Autodesk Inventor part; units mm, degrees
ref_plane "YZ Plane" through (0, 0, 0) normal (1, 0, 0) x (0, 1, 0)
ref_plane "XZ Plane" through (0, 0, 0) normal (0, 1, 0) x (-1, 0, 0)
ref_plane "XY Plane" through (0, 0, 0) normal (0, 0, 1) x (1, 0, 0)
sketch "スケッチ1" plane through (0, 0, 0) normal (0, 1, 0) x (-1, 0, 0)
  line L0 (41.0243, -3.6426) -> (37.5574, -0.1757)
  line L1 (41.0243, -37.5574) -> (37.5574, -41.0243)
  line L2 (3.6426, -0.1757) -> (0.1757, -3.6426)
  line L3 (0.1757, -37.5574) -> (3.6426, -41.0243)
  line L4 (0, -37.1331) -> (0, -4.0669)
  line L5 (37.1331, -41.2) -> (4.0669, -41.2)
  line L6 (41.2, -4.0669) -> (41.2, -37.1331)
  line L7 (37.1331, 0) -> (4.0669, 0)
  arc A0 (41.2, -4.0669) -> (41.0243, -3.6426) centre (40.6, -4.0669) ccw
  arc A1 (37.5574, -0.1757) -> (37.1331, 0) centre (37.1331, -0.6) ccw
  arc A2 (4.0669, 0) -> (3.6426, -0.1757) centre (4.0669, -0.6) ccw
  arc A3 (0.1757, -3.6426) -> (0, -4.0669) centre (0.6, -4.0669) ccw
  arc A4 (0, -37.1331) -> (0.1757, -37.5574) centre (0.6, -37.1331) ccw
  arc A5 (3.6426, -41.0243) -> (4.0669, -41.2) centre (4.0669, -40.6) ccw
  arc A6 (37.1331, -41.2) -> (37.5574, -41.0243) centre (37.1331, -40.6) ccw
  arc A7 (41.0243, -37.5574) -> (41.2, -37.1331) centre (40.6, -37.1331) ccw
  line L8 (25.8, 0) -> (15.4, 0)
  point P0 (0, 0)
  point P1 (41.2, -3.8184)
  point P2 (37.3816, 0)
  point P3 (39.2908, -1.9092)
  point P4 (37.3816, -41.2)
  point P5 (41.2, -37.3816)
  dimension "d2" = 5.4
  dimension "d3" = 5.4
  dimension "d4" = 0.6
extrude "押し出し1" add sketch "スケッチ1" along normal blind 9.8
sketch "スケッチ2" plane through (0, 9.8, 0) normal (0, 1, 0) x (1, 0, 0)
  line L0 (-41.2, 37.1331) -> (-41.2, 4.0669)
  line L1 (-41.0243, 3.6426) -> (-37.5574, 0.1757)
  line L2 (-4.0669, 41.2) -> (-37.1331, 41.2)
  line L3 (0, 4.0669) -> (0, 37.1331)
  line L4 (-37.1331, 0) -> (-4.0669, 0)
  line L5 (0, 34.1568) -> (0, 7.099)
  line L6 (-7.099, 0) -> (-34.1289, 0)
  line L7 (-41.2, 7.0711) -> (-41.2, 34.1568)
  line L8 (-37.5574, 41.0243) -> (-41.0243, 37.5574)
  line L9 (-3.6426, 0.1757) -> (-0.1757, 3.6426)
  arc A0 (-41.2, 7.0711) -> (-34.1289, 0) centre (-20.6, 20.6) ccw
  arc A1 (-7.071, 0) -> (0, 7.071) centre (-20.6, 20.6) ccw
  arc A2 (0, 34.1289) -> (-7.0711, 41.2) centre (-20.6, 20.6) ccw
  arc A3 (-34.1289, 41.2) -> (-41.2, 34.1289) centre (-20.6, 20.6) ccw
  line L10 (-34.1289, 0) -> (-7.071, 0)
  line L11 (-41.2, 7.0711) -> (-41.2, 34.1289)
  line L12 (-34.1289, 41.2) -> (-7.0711, 41.2)
  line L13 (0, 34.1289) -> (0, 7.071)
  point P0 (0, 0)
  point P1 (0, 40.8633)
  point P2 (-37.6645, 3.5355)
  point P3 (0, 34.1289)
  point P4 (-41.2, 41.2)
  point P5 (-7.071, 0)
  point P6 (0, 7.071)
  dimension "d8" = 10
  dimension "d9" = 10
extrude "押し出し2" add sketch "スケッチ2" along normal blind 3.8
ref_plane "作業平面1" through (0, 13.6, 0) normal (0, 1, 0) x (1, 0, 0)
sketch "スケッチ4" plane through (0, 13.6, 0) normal (0, 1, 0) x (1, 0, 0)
  line L0 (-4.0669, 0) -> (-37.1331, 0)
  line L1 (-41.2, 4.0669) -> (-41.2, 37.1331)
  line L2 (-37.1331, 41.2) -> (-4.0669, 41.2)
  line L3 (0, 37.1331) -> (0, 4.0669)
  line L4 (-41.0243, 3.6426) -> (-37.5574, 0.1757)
  line L5 (-41.0243, 3.6426) -> (-37.5574, 0.1757)
  line L6 (-0.1757, 37.5574) -> (-3.6426, 41.0243)
  line L7 (-3.6426, 41.0243) -> (-0.1757, 37.5574)
  line L8 (-3.6426, 0.1757) -> (-0.1757, 3.6426)
  line L9 (-0.1757, 3.6426) -> (-3.6426, 0.1757)
  line L10 (-37.5574, 41.0243) -> (-41.0243, 37.5574)
  line L11 (-37.5574, 41.0243) -> (-41.0243, 37.5574)
  arc A0 (-37.1331, 41.2) -> (-37.5574, 41.0243) centre (-37.1331, 40.6) ccw
  arc A1 (-41.0243, 37.5574) -> (-41.2, 37.1331) centre (-40.6, 37.1331) ccw
  line L12 (-41.0243, 3.6426) -> (-37.5574, 0.1757)
  arc A2 (-41.2, 4.0669) -> (-41.0243, 3.6426) centre (-40.6, 4.0669) ccw
  arc A3 (-37.5574, 0.1757) -> (-37.1331, 0) centre (-37.1331, 0.6) ccw
  arc A4 (-3.6426, 41.0243) -> (-4.0669, 41.2) centre (-4.0669, 40.6) ccw
  arc A5 (0, 37.1331) -> (-0.1757, 37.5574) centre (-0.6, 37.1331) ccw
  line L13 (-0.1757, 3.6426) -> (-3.6426, 0.1757)
  arc A6 (-0.1757, 3.6426) -> (0, 4.0669) centre (-0.6, 4.0669) ccw
  arc A7 (-4.0669, 0) -> (-3.6426, 0.1757) centre (-4.0669, 0.6) ccw
  point P0 (0, 0)
  point P1 (-41.2, 41.2)
  point P2 (-41.2, 0)
  point P3 (0, 41.2)
  point P4 (-41.0243, 37.5574)
  point P5 (-0.1757, 3.6426)
  dimension "d16" = 41.2
  dimension "d17" = 41.2
  dimension "d18" = 0.6
  dimension "d19" = 0.6
  dimension "d20" = 0.6
  dimension "d21" = 0.6
  dimension "d22" = 0.6
extrude "押し出し3" add sketch "スケッチ4" along normal blind 9.8
ref_plane "作業平面2" through (0, 0, 0) normal (0, -1, 0) x (1, 0, 0)
sketch "スケッチ5" plane through (0, 0, 0) normal (0, -1, 0) x (1, 0, 0)
  line L0 (-37.1331, 0) -> (-4.0669, 0)
  line L1 (-37.1331, 0) -> (-4.0669, 0)
  line L2 (-28.3, 0) -> (-12.9, 0)
  line L3 (-12.9, 0) -> (-12.9, 3.9)
  line L4 (-13, 4) -> (-28.2, 4)
  line L5 (-28.3, 3.9) -> (-28.3, 0)
  arc A0 (-28.2, 4) -> (-28.3, 3.9) centre (-28.2, 3.9) ccw
  arc A1 (-12.9, 3.9) -> (-13, 4) centre (-13, 3.9) ccw
  point P0 (0, 0)
  point P1 (-15.4, 0)
  point P2 (-12.9, 4)
  point P3 (-28.3, 4)
  point P4 (-28.3, 0)
  point P5 (-12.9, 0)
  point P6 (-20.6, 0)
  point P7 (-20.6, 0)
  dimension "d35" = 0.1
  dimension "d77" = 15.4
extrude "押し出し4" add sketch "スケッチ5" against normal blind 2
fillet "フィレット1" radius 0.1 5 edges at (-12.9, 2, 1.95) (-20.6, 2, 4) (-28.2707, 2, 3.9707) (-28.3, 2, 1.95) (-12.9293, 2, 3.9707)
ref_plane "作業平面3" through (0, 23.4, 0) normal (0, 1, 0) x (1, 0, 0)
sketch "スケッチ6" plane through (0, 23.4, 0) normal (0, 1, 0) x (1, 0, 0)
  line L0 (-41.2, 37.1331) -> (-41.2, 4.0669)
  line L1 (-4.0669, 41.2) -> (-37.1331, 41.2)
  line L2 (0, 4.0669) -> (0, 37.1331)
  line L3 (-37.1331, 0) -> (-4.0669, 0)
  circle A0 centre (-36.1, 5.1) radius 1.5
  circle A1 centre (-36.1, 36.1) radius 1.5
  circle A2 centre (-5.1, 36.1) radius 1.5
  circle A3 centre (-5.1, 5.1) radius 1.5
  point P0 (0, 0)
  dimension "d39" = 5.1
  dimension "d40" = 5.1
  dimension "d41" = 5.1
  dimension "d42" = 5.1
  dimension "d43" = 5.1
  dimension "d44" = 5.1
  dimension "d45" = 5.1
  dimension "d46" = 5.1
  dimension "d47" = 3
  dimension "d48" = 3
  dimension "d49" = 3
  dimension "d50" = 3
hole "穴1" at (-36.1, 23.4, -5.1) at (-36.1, 23.4, -36.1) at (-5.1, 23.4, -36.1) at (-5.1, 23.4, -5.1) direction (0, -1, 0) diameter 3 depth 4.5
sketch "スケッチ7" plane through (0, 23.4, 0) normal (0, 1, 0) x (1, 0, 0)
  circle A0 centre (-20.6, 20.6) radius 11
  circle A1 centre (-20.6, 20.6) radius 4.9
  point P0 (0, 0)
  dimension "d58" = 22
  dimension "d59" = 9.8
extrude "押し出し5" add sketch "スケッチ7" along normal blind 2
sketch "スケッチ8" plane through (-20.6, 23.4, -20.6) normal (0, 1, 0) x (1, 0, 0)
  circle A0 centre (0, 0) radius 4.9
  circle A1 centre (0, 0) radius 2.5
  point P0 (20.6, -20.6)
  dimension "d62" = 5
extrude "押し出し6" add sketch "スケッチ8" along normal blind 5.6 contours A1
ref_plane "作業平面4" through (-20.6, 29, -20.6) normal (0, 1, 0) x (1, 0, 0)
sketch "スケッチ9" plane through (-20.6, 29, -20.6) normal (0, 1, 0) x (1, 0, 0)
  line L0 (-1.8244, 1.7093) -> (1.1301, 2.23)
  circle A0 centre (0, 0) radius 2.5
  arc A1 (-1.8244, 1.7093) -> (1.1301, 2.23) centre (0, 0) ccw
  point P0 (20.6, -20.6)
  dimension "d67" = 3
extrude "押し出し7" add sketch "スケッチ9" along normal blind 17.4 contours L0 A0 picked at (-1.0191, 0.489)
fillet "フィレット2" radius 0.1 1 edges at (-20.1661, 46.4, -18.1379)
ref_plane "作業平面5" through (0, 2.3, 0) normal (0, 1, 0) x (1, 0, 0)
sketch "スケッチ10" plane through (0, 2.3, 0) normal (0, 1, 0) x (1, 0, 0)
  line L0 (-37.1331, 0) -> (-4.0669, 0)
  line L1 (-28.15, 0) -> (-13.05, 0)
  line L2 (-13.05, 0) -> (-13.05, -5)
  line L3 (-13.05, -5) -> (-28.15, -5)
  line L4 (-28.15, -5) -> (-28.15, 0)
  point P0 (0, 0)
  point P1 (-13.05, 0)
  point P2 (-13.05, 0)
  dimension "d74" = 5
  dimension "d80" = 15.1
extrude "押し出し8" add sketch "スケッチ10" along normal blind 6
sketch "スケッチ11" plane through (0, 0, 0) normal (0, -1, 0) x (1, 0, 0)
  circle A0 centre (-20.6, -20.6) radius 5
  point P0 (0, 0)
  dimension "d81" = 10
hole "穴2" at (-20.6, 0, -20.6) direction (0, 1, 0) diameter 10 depth 3
properties part number "stepper_motor"
CAD build for the part. Positions are in the model's coordinates, mm. A direction names the side the tool comes from. Round coordinates to 2 decimals unless told otherwise and drop trailing zeros. Loops run counter-clockwise (first coordinate to the right, second up) from the corner with the lowest first, then second, coordinate; pieces in that order, holes last. Notation, with made-up numbers: M 75.5,-29.75 L 100.5,-29.75 A4 ccw 100.5,-23.75 Z; hole C 20.25,45.25 d11. An arc over 180 degrees is marked long. Return JSON: item names as keys, results as strings. Group by question number.
(1) Saw through at C-C, the plane x = -27.5. List the corners of the cut face in (y, z).
(2) Saw through at B-B, the plane z = -36.1. List the corners of the cut face in (x, y), and give its area (3 significant figures).
(3) Mould opens along Z. For faces 4 (the flat face through (-36, 18.9, -36)), 5 (the flat face through (-20, 1, 4)), 6 (the flat face through (0, 12, -21)), 7 (the flat face through (-36, 18.9, -5)) say: +Z half, -Z half, draft (parallel to the pull), parting line (faces both ways), or undercut.
(4) Wall check: probe 1 along Z at (x, y) = (-5.1, 20.55); probe 2 along X at (y, z) = (24.85, -20.6). Give the ranges that are in metal, low to high. Write a range as [from, to].
(5) Saw through at A-A, the plane y = 18. List the corners of the cut face in (x, z), and give its area (3 significant figures).
(6) Tool access for faces 1 (the flat face through (-12.9, 1, 2)), 2 (the flat face through (-13.05, 5, 2)), 3 (the flat face through (-39, 13.6, -39)): list every direction of +Z, -Z, +X, -X, +Y, -Y with a clear straight run to the whole face (end or side of a thin tool).
(7) Saw through at D-D, the plane z = -30.5. List the corners of the cut face in (x, y), and give its area (3 significant figures).
(8) Drop flat-ended pins along their axis: P1, Ø4, axis at x = -5.1, z = -5.1, coming from the -Y side; P2, Ø3.5, axis at x = -36, z = -35.5, coming from the +Y side; P3, Ø1, axis at x = -27.5, y = 12, coming from the +Z side; P4, Ø1.2, axis at x = -20.5, z = 2, coming from the +Y side. Give the stop position or say it passes through.
Answer list:
{
 "1": {"outline": "M 0,-41.2 L 23.4,-41.2 L 23.4,-29.17 L 25.4,-29.17 L 25.4,-12.03 L 23.4,-12.03 L 23.4,0 L 8.3,0 L 8.3,5 L 2.3,5 L 2.3,0 L 2,0 L 2,3.9 A0.1 ccw 1.9,4 L 0,4 Z"},
 "2": {"outline": "M -41.2,0 L 0,0 L 0,9.8 L -1.44,9.8 L -1.44,13.6 L 0,13.6 L 0,23.4 L -3.6,23.4 L -3.6,18.9 L -6.6,18.9 L -6.6,23.4 L -34.6,23.4 L -34.6,18.9 L -37.6,18.9 L -37.6,23.4 L -41.2,23.4 L -41.2,13.6 L -39.76,13.6 L -39.76,9.8 L -41.2,9.8 Z", "area": "926 mm2"},
 "3": {"face 4": "undercut", "face 5": "+Z half", "face 6": "draft", "face 7": "undercut"},
 "4": {"probe 1": "[-41.2, -37.6], [-34.6, -6.6], [-3.6, 0]", "probe 2": "[-31.6, -25.5], [-23.1, -18.1], [-15.7, -9.6]"},
 "5": {"outline": "M -41.2,-37.13 A0.6 ccw -41.02,-37.56 L -37.56,-41.02 A0.6 ccw -37.13,-41.2 L -4.07,-41.2 A0.6 ccw -3.64,-41.02 L -0.18,-37.56 A0.6 ccw 0,-37.13 L 0,-4.07 A0.6 ccw -0.18,-3.64 L -3.64,-0.18 A0.6 ccw -4.07,0 L -37.13,0 A0.6 ccw -37.56,-0.18 L -41.02,-3.64 A0.6 ccw -41.2,-4.07 Z", "area": "1,670 mm2"},
 "6": {"face 1": "+Z, +X, +Y, -Y", "face 2": "+Z, +X, +Y", "face 3": "-Z, -X"},
 "7": {"outline": "M -41.2,0 L 0,0 L 0,23.4 L -15.81,23.4 L -15.81,25.4 L -25.39,25.4 L -25.39,23.4 L -41.2,23.4 Z", "area": "983 mm2"},
 "8": {"P1": "y = 0", "P2": "y = 23.4", "P3": "z = 0", "P4": "y = 8.3"}
}
